The model under review builds one solid part; all positions refer to its coordinate system, in mm. A direction names the side the tool comes from. Round coordinates to 2 decimals unless told otherwise and drop trailing zeros. Loops run counter-clockwise (first coordinate to the right, second up) from the corner with the lowest first, then second, coordinate; pieces in that order, holes last. Notation, with made-up numbers: M -7.75,51 L 8.25,51 A15 ccw 8.25,72 Z; hole C -19,7.25 d3. An arc over 180 degrees is marked long. Answer as a JSON object with one key per item and string values. Group by question number.
Item 1: Consider section A-A (x = -82.5). Give the boundary of the cut face in (y, z).
Item 2: To check wall thickness, follow line 1 (X direction, y = -26, z = 104); line 2 (Y direction, x = -126.5, z = -135.5); line 3 (Z direction, x = 8, y = -100.5). State the ranges of each line that lie inside material, in increasing order.
Item 3: Consider section D-D (y = -22). Give the boundary of the cut face in (x, z), and give its area (3 significant figures).
Item 4: Tool access review of faces 5 (the face through (-54, -175, 2)), 6 (the face through (-54, -89, -152.164)): name each direction out of +Z, -Z, +X, -X, +Y, -Y from which nothing blocks a thin tool from reaching the whole face with its end or side.
Item 5: The part is to be moulded in two halves that separate along Y. For faces 1 (the face through (-54, -5, 2)), 2 (the face through (-54, 0, 0)), 3 (the face through (-54, -180, 0)), 4 (the face through (37.05, -89, -4)), say which applies: +Y half, -Y half, draft (parallel to the pull), parting line (faces both ways), or undercut.
Item 6: Consider section C-C (x = -129.5). Give the boundary of the cut face in (y, z).
Item 7: Consider section B-B (z = -44). State how many separate pieces and enclosed holes the cut face has, and give its area (3 significant figures).
Item 8: Insertion check: P1, Ø1.5, axis at x = -93, y = -65, coming from the +Z side. The pin has a flat end and moves straight along its axis. Give the tip position at first contact, or say it passes through.
```python
from build123d import *

# Parameters (mm, degrees)
F0_W     = 180
F0_H     = 300
F1_DEPTH = 180
F2_T     = -5
F3_W     = 15
F3_H     = 210.58443
F3_W_2   = 9.852498
F3_W_3   = 9.454142
F3_W_4   = 9.030989
F3_W_5   = 11.25
F4_DEPTH = 25


with BuildPart() as f1:
    # F0 (on Front) → F1 (new body)
    with BuildSketch(Plane.XZ):
        with Locations((-52.950007, -2.163574)):
            Rectangle(F0_W, F0_H)
    extrude(amount=F1_DEPTH)

    # F2
    f2_openings = [f1.faces().sort_by_distance(p)[0] for p in [
        (-52.950007, -90, 147.836426),
    ]]
    offset(amount=F2_T, openings=f2_openings)

    # F3 (on face) → F4 (cut)
    with BuildSketch(Plane.XZ.offset(180)):
        with Locations((-116.25, 22.645805)):
            Rectangle(F3_W, F3_H)
        with Locations((-98.676249, 22.645805)):
            Rectangle(F3_W_2, F3_H)
        with Locations((-81.25, 22.645805)):
            Rectangle(F3_W, F3_H)
        with Locations((-63.477071, 22.645805)):
            Rectangle(F3_W_3, F3_H)
        with Locations((-46.25, 22.645808)):
            Rectangle(F3_W, F3_H)
        with Locations((-28.265494, 22.645808)):
            Rectangle(F3_W_4, F3_H)
        with Locations((-11.25, 22.645808)):
            Rectangle(F3_W, F3_H)
        with Locations((5.625, 22.645808)):
            Rectangle(F3_W_5, F3_H)
    extrude(amount=-F4_DEPTH, mode=Mode.SUBTRACT)


solid = f1.part
```
Geometry results:
{
 "1": {"outline": "M -180,-152.16 L 0,-152.16 L 0,147.84 L -5,147.84 L -5,-147.16 L -175,-147.16 L -175,-82.65 L -180,-82.65 Z; M -180,127.94 L -175,127.94 L -175,147.84 L -180,147.84 Z"},
 "2": {"line 1": "x = -142.95 to -137.95, 32.05 to 37.05", "line 2": "y = -180 to -175, -5 to 0", "line 3": "z = -152.16 to -147.16"},
 "3": {"outline": "M -142.95,-152.16 L 37.05,-152.16 L 37.05,147.84 L 32.05,147.84 L 32.05,-147.16 L -137.95,-147.16 L -137.95,147.84 L -142.95,147.84 Z", "area": "3,850 mm^2"},
 "4": {"face 5": "+Z", "face 6": "-Z, +X, -X, +Y, -Y"},
 "5": {"face 1": "undercut", "face 2": "+Y half", "face 3": "-Y half", "face 4": "draft"},
 "6": {"outline": "M -180,-152.16 L 0,-152.16 L 0,147.84 L -5,147.84 L -5,-147.16 L -175,-147.16 L -175,147.84 L -180,147.84 Z"},
 "7": {"separate pieces": "8", "enclosed holes": "0", "area": "3,000 mm^2"},
 "8": {"P1": "stops at z = -147.16"}
}
